```python
from build123d import *

# Parameters (mm, degrees)
SKETCH2_R           = 12.02
SKETCH2_R_2         = 10.75
BOSS_EXTRUDE1_DEPTH = 19.3
SKETCH3_R           = 3.6
BOSS_EXTRUDE4_DEPTH = 1.27
BOSS_EXTRUDE5_DEPTH = 6.02
BOSS_EXTRUDE6_DEPTH = 19.3
CUT_EXTRUDE1_DEPTH  = 26
SKETCH7_R           = 1.27
CUT_EXTRUDE2_DEPTH  = 31.06


with BuildPart() as part:
    # Sketch2 → Boss-Extrude1 (new body)
    with BuildSketch(Plane.XY):
        Circle(SKETCH2_R)
        Circle(SKETCH2_R_2, mode=Mode.SUBTRACT)
    extrude(amount=BOSS_EXTRUDE1_DEPTH)

    # Sketch3 → Boss-Extrude4 (add)
    with BuildSketch(Plane.XY.offset(19.3)):
        with BuildLine():
            Line((-6.5, -6.229967897), (-6.5, 6.229967897))
            ThreePointArc((-6.5, 6.229967897), (-7.16031689, 7.17050784), (-8.269230769, 6.868938964))
            ThreePointArc((-8.269230769, 6.868938964), (0, 10.75), (8.269230769, 6.868938964))
            ThreePointArc((8.269230769, 6.868938964), (7.16031689, 7.17050784), (6.5, 6.229967897))
            Line((6.5, 6.229967897), (6.5, -6.229967897))
            ThreePointArc((6.5, -6.229967897), (7.16031689, -7.17050784), (8.269230769, -6.868938964))
            ThreePointArc((8.269230769, -6.868938964), (0, -10.75), (-8.269230769, -6.868938964))
            ThreePointArc((-8.269230769, -6.868938964), (-7.16031689, -7.17050784), (-6.5, -6.229967897))
        make_face()
        Circle(SKETCH3_R, mode=Mode.SUBTRACT)
    extrude(amount=-BOSS_EXTRUDE4_DEPTH)



with BuildPart() as body_2:
    # Sketch4 → Boss-Extrude5 (new body)
    with BuildSketch(Plane(origin=(0, -12.02, 0), x_dir=(1, 0, 0), z_dir=(0, 1, 0))):
        with BuildLine():
            Line((-12.02, -19.3), (12.02, -19.3))
            Line((12.02, -19.3), (16.755, -19.3))
            ThreePointArc((16.755, -19.3), (18.551051224, -18.556051224), (19.295, -16.76))
            Line((19.295, -16.76), (19.295, 3.16))
            ThreePointArc((19.295, 3.16), (18.551051224, 4.956051224), (16.755, 5.7))
            Line((16.755, 5.7), (-16.755, 5.7))
            ThreePointArc((-16.755, 5.7), (-18.551051224, 4.956051224), (-19.295, 3.16))
            Line((-19.295, 3.16), (-19.295, -16.76))
            ThreePointArc((-19.295, -16.76), (-18.551051224, -18.556051224), (-16.755, -19.3))
            Line((-16.755, -19.3), (-12.02, -19.3))
        make_face()
    extrude(amount=-BOSS_EXTRUDE5_DEPTH)


with BuildPart() as part_1:
    add(part.part)

    add(body_2.part)  # Boss-Extrude6 merges body 2
    # Sketch5 → Boss-Extrude6 (add)
    with BuildSketch(Plane.XY.offset(19.3)):
        with BuildLine():
            Line((-10, -12.02), (-11.050936612, -12.02))
            ThreePointArc((-11.050936612, -12.02), (-8.743098915, -10.540888856), (-9.123094648, -7.826208791))
            ThreePointArc((-9.123094648, -7.826208791), (0, -12.02), (9.123094648, -7.826208791))
            ThreePointArc((9.123094648, -7.826208791), (8.743098915, -10.540888856), (11.050936612, -12.02))
            Line((11.050936612, -12.02), (10, -12.02))
            Line((10, -12.02), (10, -18.04))
            Line((10, -18.04), (-10, -18.04))
            Line((-10, -18.04), (-10, -12.02))
        make_face()
    extrude(amount=-BOSS_EXTRUDE6_DEPTH)

    # Sketch6 → Cut-Extrude1 (cut, through all)
    with BuildSketch(Plane.XY.offset(19.3)):
        with BuildLine():
            Line((-8.89, -18.04), (-8.89, -14.74))
            ThreePointArc((-8.89, -14.74), (-8.597106781, -14.032893219), (-7.89, -13.74))
            Line((-7.89, -13.74), (-4.81, -13.74))
            ThreePointArc((-4.81, -13.74), (-4.102893219, -14.032893219), (-3.81, -14.74))
            Line((-3.81, -14.74), (-3.81, -18.04))
            Line((-3.81, -18.04), (-8.89, -18.04))
        make_face()
        with BuildLine():
            Line((3.81, -14.74), (3.81, -18.04))
            Line((3.81, -18.04), (8.89, -18.04))
            Line((8.89, -18.04), (8.89, -14.74))
            ThreePointArc((8.89, -14.74), (8.597106781, -14.032893219), (7.89, -13.74))
            Line((7.89, -13.74), (4.81, -13.74))
            ThreePointArc((4.81, -13.74), (4.102893219, -14.032893219), (3.81, -14.74))
        make_face()
    extrude(amount=-CUT_EXTRUDE1_DEPTH, mode=Mode.SUBTRACT)

    # Sketch7 → Cut-Extrude2 (cut, through all)
    with BuildSketch(Plane.XZ.offset(18.04)):
        with Locations((-15.485, 14.22)):
            Circle(SKETCH7_R)
        with Locations((15.485, 14.22)):
            Circle(SKETCH7_R)
        with Locations((-15.485, -0.62)):
            Circle(SKETCH7_R)
        with Locations((15.485, -0.62)):
            Circle(SKETCH7_R)
    extrude(amount=-CUT_EXTRUDE2_DEPTH, mode=Mode.SUBTRACT)


solid = part_1.part
```
The listing builds one solid part. Answer for the finished solid, in the listing's coordinates (mm). A direction names the side the tool comes from. Give positions to 0.01 mm unless a question says otherwise; leave off trailing zeros. Write each loop counter-clockwise with the first axis right and the second up, starting at its lowest first coordinate (ties: lowest second). Pieces come first, ordered by that corner, then holes. Notation, with made-up numbers: M 66,-5.5 L 87,-5.5 A16 cw 87,21.5 Z; hole C -16,-35 d6. An arc over 180 degrees is marked long. Write each question's results on one line, items separated by ' | '.
Q1. Flat-ended cylindrical pins translate along their axes: P1, Ø3, axis at x = -6.5, z = 15.5, coming from the +Y side; P2, Ø7, axis at x = -4.5, y = 1, coming from the -Z side; P3, Ø1, axis at y = 0, z = 18.5, coming from the +X side; P4, Ø1, axis at y = -12, z = 1, coming from the -X side (3 decimals). Find the tip coordinate at first contact, or state that the pin passes through.
Output values:
P1: y = 10.93 | P2: z = 18.03 | P3: x = 12.02 | P4: x = -19.295
Q2. A tool of negligible diameter and unlimited length cuts with its end or side. For faces 4 (the flat face through (6.5, 0, 19)), 5 (the flat face through (-19.295, -15, 7)), 6 (the flat face through (-2, -11, 0)), 7 (the cylindrical face through (-18.571, -14.988, 18.536)), 8 (the flat face through (6, -13.74, 7)), from which of +Z, -Z, +X, -X, +Y, -Y can it reach the whole face along a straight path? Write none if from no direction.
Output values:
face 4: +Z, -Z | face 5: +Z, -Z, -X, +Y, -Y | face 6: -Z, +X, -X, +Y | face 7: +Z, -X, +Y, -Y | face 8: +Z, -Z, -Y
Q3. Section C-C, the plane x = -3 is taken. Write down the section's boundary in (y, z), then the cut area to 3 significant figures.
Output values:
outline: M -18.04,-5.7 L -12.02,-5.7 L -12.02,0 L -10.32,0 L -10.32,18.03 L -1.99,18.03 L -1.99,19.3 L -18.04,19.3 Z; M 1.99,18.03 L 10.32,18.03 L 10.32,0 L 11.64,0 L 11.64,19.3 L 1.99,19.3 Z | area: 230 mm2
Q4. Consider L1, parallel to X at y = -13.5, z = -1.25 (3 decimals); L2, parallel to X at y = 0, z = 8.75; L3, parallel to Y at x = 0.5, z = 4.5. Determine where each line is inside the solid, lowest interval first. Write a range as from..to.
Output values:
L1: -19.295..-16.588, -14.382..14.382, 16.588..19.295 | L2: -12.02..-10.75, 10.75..12.02 | L3: -18.04..-10.74, 10.74..12.01
Q5. Section A-A, the plane y = 0 is taken. Write down the section's boundary in (x, z).
Output values:
outline: M -12.02,0 L -10.75,0 L -10.75,19.3 L -12.02,19.3 Z; M -6.5,18.03 L -3.6,18.03 L -3.6,19.3 L -6.5,19.3 Z; M 3.6,18.03 L 6.5,18.03 L 6.5,19.3 L 3.6,19.3 Z; M 10.75,0 L 12.02,0 L 12.02,19.3 L 10.75,19.3 Z
Q6. For a pull along Y with two mould halves and no side action, classify faces 1 (the cylindrical face through (-7.144, 7.165, 18.674)), 2 (the flat face through (-8.89, -16, 7)), 3 (the cylindrical face through (-4.111, -14.025, 6.975)) as released by +Y, released by -Y, zero draft, split by the parting line, or undercut.
Output values:
face 1: undercut | face 2: zero draft | face 3: released by -Y
Q7. Section D-D, the plane z = -0.62 is taken. Write down the section's boundary in (x, y) (3 decimals), then the cut area to 3 significant figures.
Output values:
outline: M -19.295,-18.04 L -16.755,-18.04 L -16.755,-12.02 L -19.295,-12.02 Z; M -14.215,-18.04 L -8.89,-18.04 L -8.89,-14.74 A1 cw -7.89,-13.74 L -4.81,-13.74 A1 cw -3.81,-14.74 L -3.81,-18.04 L 3.81,-18.04 L 3.81,-14.74 A1 cw 4.81,-13.74 L 7.89,-13.74 A1 cw 8.89,-14.74 L 8.89,-18.04 L 14.215,-18.04 L 14.215,-12.02 L -14.215,-12.02 Z; M 16.755,-18.04 L 19.295,-18.04 L 19.295,-12.02 L 16.755,-12.02 Z | area: 159 mm2
Q8. Section B-B, the plane z = 14.22 is taken. Count the separate pieces of the cut face and the enclosed holes in it, then the cut area to 3 significant figures.
Output values:
separate pieces: 3 | enclosed holes: 1 | area: 271 mm2
